Autodesk Inventor part; units mm, degrees
ref_plane "YZ Plane" through (0, 0, 0) normal (1, 0, 0) x (0, 1, 0)
ref_plane "XZ Plane" through (0, 0, 0) normal (0, 1, 0) x (-1, 0, 0)
ref_plane "XY Plane" through (0, 0, 0) normal (0, 0, 1) x (1, 0, 0)
sketch "Sketch1" plane through (0, 0, 0) normal (0, 1, 0) x (-1, 0, 0)
  arc A0 (-0.4144, 9.491) -> (0.4144, 9.491) centre (0, 0) ccw
  arc A1 (-0.4667, 10.6898) -> (0.4667, 10.6898) centre (0, 0) ccw
  line L0 (0, 0) -> (-0.4667, 10.6898)
  line L1 (0, 0) -> (0.4667, 10.6898)
  line L2 (0, 0) -> (0, 8.5605) construction
  dimension "d0" = 19
  dimension "d1" = 21.4
  dimension "d2" = 5
  dimension "d3" = 2.5
extrude "BearingSleeve" add sketch "Sketch1" along normal blind 80 contours A0 L1 A1 L0
sketch "Sketch2" plane through (0, 80, 0) normal (0, 1, 0) x (1, 0, 0)
  arc A0 (0.4144, -9.491) -> (-0.4144, -9.491) centre (0, 0) ccw
  line L0 (-0.4144, -9.491) -> (-0.816, -18.6898)
  line L1 (0.4144, -9.491) -> (0.816, -18.6898)
  line L2 (-0.4667, -10.6898) -> (-0.4144, -9.491)
  line L3 (0.4144, -9.491) -> (0.4667, -10.6898)
  line L4 (3.3903, -8.8744) -> (3.8189, -18.6898)
  line L5 (-3.3903, -8.8744) -> (-3.8189, -18.6898)
  line L6 (-3.8189, -18.6898) -> (-0.816, -18.6898)
  line L7 (0.816, -18.6898) -> (3.8189, -18.6898)
  dimension "d6" = 3
  dimension "d7" = 3
  dimension "d8" = 8
  dimension "d9" = 8
extrude "BearingLocks" add sketch "Sketch2" against normal up to surface (80 mm away)
sketch "Sketch3" plane through (-3.4452, 0, 10.1302) normal (-0.9990482, 0, -0.0436194) x (-0.0436194, 0, 0.9990482)
  line L0 (8.5678, 0) -> (0, 0)
  line L1 (0, 80) -> (8.5678, 80)
  line L2 (8.5678, 80) -> (8.5678, 0)
  point P0 (-10.2708, 0)
  point P1 (4.1678, 14.5)
  point P2 (4.1678, 65.5)
  dimension "d12" = 14.5
  dimension "d13" = 14.5
  dimension "d14" = 4.4
  dimension "d15" = 4.4
hole "Hole1" at (-3.6269, 14.5, 14.294) at (-3.6269, 65.5, 14.294) direction (0.9990482, 0, 0.0436194) diameter 3.6 end up to surface counterbore diameter 6.5 counterbore depth 1.5
sketch "Sketch4" plane through (3.4452, 0, 10.1302) normal (0.9990482, 0, -0.0436194) x (-0.0436194, 0, -0.9990482)
  line L0 (-8.5678, 80) -> (0, 80)
  line L1 (0, 0) -> (-8.5678, 0)
  line L2 (-8.5678, 80) -> (-8.5678, 0)
  point P0 (10.2708, 0)
  point P1 (-4.1678, 65.5)
  point P2 (-4.1678, 14.5)
  dimension "d23" = 14.5
  dimension "d24" = 14.5
  dimension "d25" = 4.4
  dimension "d26" = 4.4
hole "Hole2" at (3.6269, 65.5, 14.294) at (3.6269, 14.5, 14.294) direction (-0.9990482, 0, 0.0436194) diameter 3.4 depth 3
sketch "Sketch5" plane through (3.4452, 0, 10.1302) normal (0.9990482, 0, -0.0436194) x (-0.0436194, 0, -0.9990482)
  circle A0 centre (-4.1678, 65.5) radius 1.7
  circle A1 centre (-4.1678, 14.5) radius 1.7
  line L0 (0, 80) -> (0, 0)
  line L1 (-8.5678, 80) -> (0, 80)
  line L2 (-8.5678, 80) -> (-8.5678, 0)
  line L3 (0, 0) -> (-8.5678, 0)
  line L4 (-1.4178, 12.9123) -> (-4.1678, 11.3246)
  line L5 (-4.1678, 11.3246) -> (-6.9178, 12.9123)
  line L6 (-6.9178, 12.9123) -> (-6.9178, 16.0877)
  line L7 (-6.9178, 16.0877) -> (-4.1678, 17.6754)
  line L8 (-4.1678, 17.6754) -> (-1.4178, 16.0877)
  line L9 (-1.4178, 16.0877) -> (-1.4178, 12.9123)
  line L10 (-1.4178, 63.9123) -> (-4.1678, 62.3246)
  line L11 (-4.1678, 62.3246) -> (-6.9178, 63.9123)
  line L12 (-6.9178, 63.9123) -> (-6.9178, 67.0877)
  line L13 (-6.9178, 67.0877) -> (-4.1678, 68.6754)
  line L14 (-4.1678, 68.6754) -> (-1.4178, 67.0877)
  line L15 (-1.4178, 67.0877) -> (-1.4178, 63.9123)
  point P0 (10.2708, 0)
  dimension "d34" = 5.5
  dimension "d35" = 5.5
extrude "Extrusion3" cut sketch "Sketch5" against normal blind 2 contours L4 L5 L6 L7 L8 L9 | L10 L11 L12 L13 L14 L15
equation "\"d0\" = BearingOD"
equation "\"d1\" = BearingOD + BearingClampWallThickness"
equation "\"d2\" = BearingTensionGap"
equation "\"d3\" = 0.5 * BearingTensionGap"
equation "\"d4\" = EffectiveBearingLength"
equation "\"d10\" = EffectiveBearingLength"
equation "\"BearingOD\" = 19"
equation "\"NozzleDiameter\" = 0.4"
equation "\"BearingTensionGap\" = 5deg"
equation "\"BearingLength\" = 29"
equation "\"EffectiveBearingLength\" = 80"
equation "\"BearingSpacing\" = EffectiveBearingLength - 2 * BearingLength"
equation "\"BearingClampWallThickness\" = 6 * NozzleDiameter"
equation "\"BearingClampLength\" = 8"
properties part number "X-Motor P1"
CAD build for the part. Positions are in the model's coordinates, mm. A direction names the side the tool comes from. Round coordinates to 2 decimals unless told otherwise and drop trailing zeros. Order: outer loops, then holes, each group sorted by start corner. A loop starts at its lowest first (then second) coordinate and runs counter-clockwise, first axis right, second up. Notation, with made-up numbers: (77, 50.5) - (88, 50.5) arc R30 cw to (88, 85.5) - close; hole circle Ø7 at (-30, -13.75). An arc over 180 degrees is marked (long way). Return JSON: item names as keys, results as strings.
(1) Pin check, flat tips, straight feed: pin 1 Ø1.5 at (y, z) = (53.5, -7) entering from -X; pin 2 Ø10 at (y, z) = (69, 12) entering from -X; pin 3 Ø1.5 at (x, z) = (7.5, 1) entering from +Y. Stop position of each tip, or through.
Answer key:
{"pin 1": "stops at x = -8.68", "pin 2": "stops at x = -8.09", "pin 3": "passes through"}
(2) Tool access for faces 1 (the face through (2.761, 14.478, 17.084)), 2 (the face through (2, 41, 18.69)), 3 (the face through (3.63, 40.56, 14.35)): list every direction of +Z, -Z, +X, -X, +Y, -Y with a clear straight run to the whole face (end or side of a thin tool).
Answer key:
{"face 1": "none", "face 2": "+Z, +X, -X, +Y, -Y", "face 3": "+X, +Y, -Y"}
(3) Cut at C-C (y = 34.5). Give the cut face in (x, z), then the cut area to 3 significant figures.
Answer key:
{"outline": "(-3.82, 18.69) - (-3.45, 10.13) arc R10.7 ccw (long way) to (3.45, 10.13) - (3.82, 18.69) - (0.82, 18.69) - (0.47, 10.69) - (0.41, 9.49) arc R9.5 cw (long way) to (-0.41, 9.49) - (-0.47, 10.69) - (-0.82, 18.69) - close", "area": "124 mm^2"}
(4) Cut at B-B (x = 8). Give the cut face in (y, z), then the cut area to 3 significant figures.
Answer key:
{"outline": "(0, -7.11) - (80, -7.11) - (80, -5.12) - (0, -5.12) - close; (0, 5.12) - (80, 5.12) - (80, 7.11) - (0, 7.11) - close", "area": "317 mm^2"}
(5) Pull direction Z, two halves, no side cores. Call faces 4 (the face through (-2, 41, 18.69)), 5 (the face through (-1, 80, 10)), 6 (the face through (2.761, 65.478, 17.084)): +Z half, -Z half, draft (parallel to the pull), parting line (faces both ways), or undercut.
Answer key:
{"face 4": "+Z half", "face 5": "draft", "face 6": "undercut"}
(6) Wall check: probe 1 along X at (y, z) = (34.5, 0); probe 2 along Z at (x, y) = (-0.25, 13.5); probe 3 along Z at (x, y) = (8, 15). Give the ranges that are in metal, low to high. Write a range as from..to.
Answer key:
{"probe 1": "x = -10.7..-9.5, 9.5..10.7", "probe 2": "z = -10.7..-9.5", "probe 3": "z = -7.11..-5.12, 5.12..7.11"}
(7) Cut at A-A (z = 0). Give the cut face in (x, y), then the cut area to 3 significant figures.
Answer key:
{"outline": "(-10.7, 0) - (-9.5, 0) - (-9.5, 80) - (-10.7, 80) - close; (9.5, 0) - (10.7, 0) - (10.7, 80) - (9.5, 80) - close", "area": "192 mm^2"}
